Source: CAD feature listing. Evaluate the final solid. Frame: model axes, mm. Face numbers are marked on the shaded views. A direction names the side the tool comes from. Coordinates: 2 decimals unless noted, no trailing zeros. Order: outer loops, then holes, each group sorted by start corner. A loop starts at its lowest first (then second) coordinate and runs counter-clockwise, first axis right, second up.
```python
from build123d import *

# Parameters (mm, degrees)
F0_R     = 44.359293
F1_DEPTH = 114.3
F2_R     = 34.168515
F3_DEPTH = 10.16
F4_R     = 34.168515
F5_DEPTH = 12.047837


with BuildPart() as f1:
    # F0 (on Top) → F1 (new body)
    with BuildSketch(Plane.XY):
        Circle(F0_R)
    extrude(amount=F1_DEPTH)

    # F2 (on face) → F3 (join)
    with BuildSketch(Plane(origin=(0, 0, 0), x_dir=(1, 0, 0), z_dir=(0, 0, -1))):
        Circle(F2_R)
    extrude(amount=F3_DEPTH)

    # F4 (on face) → F5 (join)
    with BuildSketch(Plane(origin=(0, 0, -10.16), x_dir=(1, 0, 0), z_dir=(0, 0, -1))):
        Circle(F4_R)
    extrude(amount=F5_DEPTH)


solid = f1.part
```
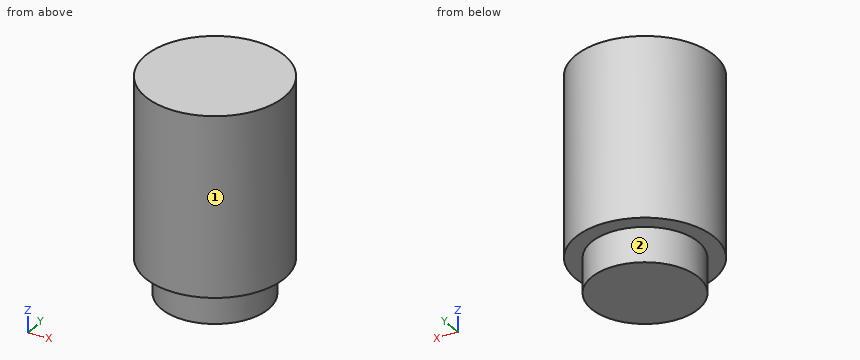
1. Section query C-C on z = -10.5. Return loops of the section in (x, y).
Findings:
outline: circle Ø68.34 at (0, 0)
2. Section query D-D on z = 65. Return loops of the section in (x, y).
Findings:
outline: circle Ø88.72 at (0, 0)
3. Ray query, line 1 (Z direction, x = -37, y = 13.5); line 2 (X direction, y = -28, z = 61.5); line 3 (X direction, y = 24.5, z = 34.5). Return the intervals inside material, ascending.
Findings:
line 1: z = 0 to 114.3
line 2: x = -34.41 to 34.41
line 3: x = -36.98 to 36.98
4. Access query for the marked faces 1 and 2. Directions: +Z, -Z, +X, -X, +Y, -Y. A direction counts if a zero-diameter tool reaches every point of the face in a straight line with its end or side. Return the directions, or none.
Findings:
face 1: +Z, -Z
face 2: -Z
5. Section query A-A on x = 0. Return loops of the section in (y, z).
Findings:
outline: (-44.36, 0) - (-34.17, 0) - (-34.17, -22.21) - (34.17, -22.21) - (34.17, 0) - (44.36, 0) - (44.36, 114.3) - (-44.36, 114.3) - close
6. Pin query (flat end, axial travel): P1, Ø3, axis at x = -33, z = 25, coming from the +Y side; P2, Ø10, axis at x = 3.5, z = 70, coming from the +Y side; P3, Ø4, axis at x = 11.5, z = 67.5, coming from the -Y side. Return the tip coordinate at first contact, or that it passes through.
Findings:
P1: stops at y = 31.23
P2: stops at y = 44.36
P3: stops at y = -43.33
